Geometry check sheet. Reference: the model listing, model coordinates, mm. Round coordinates to 2 decimals unless told otherwise and drop trailing zeros. Order: outer loops, then holes, each group sorted by start corner. A loop starts at its lowest first (then second) coordinate and runs counter-clockwise, first axis right, second up.
```python
from build123d import *

# Parameters (mm, degrees)
F0_R     = 50
F0_R_2   = 40
F1_DEPTH = 10
F5_SIZE2 = 0.5
F5_SIZE  = 1


# Not quite as in the source:
# - a pattern or mirror of a feature is missing from the dataset's text; its kind, count and spacing are read off the source's solid


with BuildPart() as f1:
    # F0 (on Top) → F1 (new body)
    with BuildSketch(Plane.XY):
        Circle(F0_R)
        Circle(F0_R_2, mode=Mode.SUBTRACT)
    extrude(amount=F1_DEPTH)

    # F2 (on Front) → F3 (revolve, cut)
    with BuildSketch(Plane.XZ):
        Polygon((-50, 13.4113135189), (-50, 10), (-47.8474881957, 10), (-47.4599111567, 9.3286968768), (-47.3599111567, 9.3286968768), (-47.2283720253, 9.5565293356), (-43.498182123, 9.5565293356), (-43.3666429916, 9.3286968768), (-43.2666429916, 9.3286968768), (-42.8790659527, 10), (-40, 10), (-40, 13.4113135189), align=None)
    f3 = revolve(axis=Axis((0, 0, 10.9280112665), (0, 0, 1)), mode=Mode.SUBTRACT)

    # F3_copies: F3 across plane
    add(f3.mirror(Plane(origin=(0, 0, 5), x_dir=(-1, 0, 0), z_dir=(0, 0, -1))), mode=Mode.SUBTRACT)

    # F5
    f5_edges = [f1.edges().sort_by_distance(p)[0] for p in [
        (-50, 0, 10),
        (-50, 0, 0),
    ]]
    f5_side = f1.faces().sort_by_distance((-50, 0, 5))[0]
    chamfer(f5_edges, length=F5_SIZE, length2=F5_SIZE2, reference=f5_side)


solid = f1.part
```
(1) Sectioned sample at A-A, the plane z = 4.75. Record the cut outline in (x, y), and give its area (3 significant figures).
Returned:
outline: circle Ø100 at (0, 0); hole circle Ø80 at (0, 0)
area: 2,830 mm2
(2) Draft check along Y on faces 1 (the cylindrical face through (47.69, 15.02, 4.94)), 2 (the flat face through (-26, 41, 10)), 3 (the cylindrical face through (-8.67, -39.05, 4.93)), 4 (the flat face through (-42, 14, 9.557)). Enter one of: released by +Y, released by -Y, zero draft, split by the parting line, or undercut.
Returned:
face 1: split by the parting line
face 2: zero draft
face 3: undercut
face 4: undercut
(3) Depth check by flat-ended pin: P1, Ø5, axis at y = 32.5, z = 3.5, coming from the +X side; P2, Ø6, axis at y = -36.5, z = 8.5, coming from the -X side; P3, Ø1, axis at y = -33, z = 5, coming from the -X side. Enter the tip coordinate at first touch or a pass-through.
Returned:
P1: stops at x = 40
P2: stops at x = -37.12
P3: stops at x = -38
(4) Material ranges on line 1 (Y direction, x = 0, z = 8); line 2 (X direction, y = 20.5, z = 9.75); line 3 (Y direction, x = -6.5, z = 0.5), recorded low to high.
Returned:
line 1: y = -50 to -40, 40 to 50
line 2: x = -45.19 to -43.07, -37.83 to -34.35, 34.35 to 37.83, 43.07 to 45.19
line 3: y = -49.32 to -47.11, -46.81 to -42.98, -42.68 to -39.47, 39.47 to 42.68, 42.98 to 46.81, 47.11 to 49.32
